Geometry check sheet. Reference: the model listing, model coordinates, mm. A direction names the side the tool comes from. Round coordinates to 2 decimals unless told otherwise and drop trailing zeros. Loops run counter-clockwise (first coordinate to the right, second up) from the corner with the lowest first, then second, coordinate; pieces in that order, holes last. Notation, with made-up numbers: (72.5, 50) -> (111.5, 50) arc R15 cw to (111.5, 70) -> close; hole circle Ø8 at (-2, -8). An arc over 180 degrees is marked (long way). Use a Markdown table: item, result. Add a question column.
Q1. Sectioned sample at D-D, the plane z = 18.5. Enter the section's corners in (x, y).
Q2. Material ranges on L1, parallel to X at y = 2.25, z = -0.5; L2, parallel to X at y = 7, z = -0.5; L3, parallel to Z at x = -19, y = 7, recorded low to high.
Q3. Release check for a two-part mould opening along X. For faces 1 (the face through (-21, 1, -28)), 2 (the face through (-23, 0, 7)), 3 (the face through (24, 6, -5)) record: released by +X, released by -X, zero draft, split by the parting line, or undercut.
Q4. Set-up check for faces 4 (the face through (5, 6, -24)), 5 (the face through (-26, 2.5, -16)): record each of +Z, -Z, +X, -X, +Y, -Y from which the full face is reachable in a straight line by a thin tool's end or side.
Q5. Sectioned sample at B-B, the plane x = 0. Enter the section's corners in (y, z), then the cut area to 3 significant figures.
Q6. Sectioned sample at C-C, the plane y = 4.25. Enter the section's corners in (x, z), then the cut area to 3 significant figures.
Q7. Gauge pin test, flat ends, axial feed: P1, Ø3.5, axis at x = -24.5, y = 5, coming from the -Z side; P2, Ø2, axis at y = 7, z = -23, coming from the -X side; P3, Ø5, axis at y = 4, z = -0.5, coming from the -X side; P4, Ø8, axis at x = 14, z = -11.5, coming from the -Y side. Record the tip position at first contact, or that the pin passes through.
Q8. Sectioned sample at A-A, the plane z = 0. Enter the section's corners in (x, y).
```python
from build123d import *

# Parameters (mm, degrees)
SKETCH1_R           = 35
SKETCH1_R_2         = 22.5
BOSS_EXTRUDE1_DEPTH = 2.5
SKETCH2_R           = 29.5
SKETCH2_R_2         = 22.5
BOSS_EXTRUDE2_DEPTH = 10
CUT_EXTRUDE1_DEPTH  = 52.051444642
SKETCH4_R           = 1.75
CUT_EXTRUDE2_DEPTH  = 52.051444642


with BuildPart() as part:
    # Sketch1 → Boss-Extrude1 (new body)
    with BuildSketch(Plane(origin=(0, 0, 0), x_dir=(1, 0, 0), z_dir=(0, 1, 0))):
        with Locations(Location((0, 0, 0), (0, 0, 270))):
            Circle(SKETCH1_R)
        with Locations(Location((0, 0, 0), (0, 0, 270))):
            Circle(SKETCH1_R_2, mode=Mode.SUBTRACT)
    extrude(amount=BOSS_EXTRUDE1_DEPTH)

    # Sketch2 → Boss-Extrude2 (add)
    with BuildSketch(Plane(origin=(0, 2.5, 0), x_dir=(1, 0, 0), z_dir=(0, 1, 0))):
        with Locations(Location((0, 0, 0), (0, 0, 270))):
            Circle(SKETCH2_R)
        with Locations(Location((0, 0, 0), (0, 0, 270))):
            Circle(SKETCH2_R_2, mode=Mode.SUBTRACT)
    extrude(amount=BOSS_EXTRUDE2_DEPTH)

    # Sketch3 → Cut-Extrude1 (cut, through all)
    with BuildSketch(Plane(origin=(0, 12.5, 0), x_dir=(1, 0, 0), z_dir=(0, 1, 0))):
        with BuildLine():
            Line((-5, 21.937410968), (-5, 26))
            Line((-5, 26), (5, 26))
            Line((5, 26), (5, 21.937410968))
            ThreePointArc((5, 21.937410968), (15.909902577, 15.909902577), (21.937410968, 5))
            Line((21.937410968, 5), (26, 5))
            Line((26, 5), (26, -5))
            Line((26, -5), (21.937410968, -5))
            ThreePointArc((21.937410968, -5), (15.909902577, -15.909902577), (5, -21.937410968))
            Line((5, -21.937410968), (5, -26))
            Line((5, -26), (-5, -26))
            Line((-5, -26), (-5, -21.937410968))
            ThreePointArc((-5, -21.937410968), (-15.909902577, -15.909902577), (-21.937410968, -5))
            Line((-21.937410968, -5), (-26, -5))
            Line((-26, -5), (-26, 5))
            Line((-26, 5), (-21.937410968, 5))
            ThreePointArc((-21.937410968, 5), (-15.909902577, 15.909902577), (-5, 21.937410968))
        make_face()
    extrude(amount=-CUT_EXTRUDE1_DEPTH, mode=Mode.SUBTRACT)

    # Sketch4 → Cut-Extrude2 (cut, through all)
    with BuildSketch(Plane(origin=(0, 12.5, 0), x_dir=(1, 0, 0), z_dir=(0, 1, 0))):
        with Locations(Location((-18.384776311, -18.384776311, 0), (0, 0, 270))):
            Circle(SKETCH4_R)
        with Locations(Location((-18.384776311, 18.384776311, 0), (0, 0, 270))):
            Circle(SKETCH4_R)
        with Locations(Location((18.384776311, 18.384776311, 0), (0, 0, 270))):
            Circle(SKETCH4_R)
        with Locations(Location((18.384776311, -18.384776311, 0), (0, 0, 270))):
            Circle(SKETCH4_R)
    extrude(amount=-CUT_EXTRUDE2_DEPTH, mode=Mode.SUBTRACT)


solid = part.part
```
Values:
| question | item | result |
|---|---|---|
| 1 | outline | (-29.71, 0) -> (-20.13, 0) -> (-20.13, 12.5) -> (-22.98, 12.5) -> (-22.98, 2.5) -> (-29.71, 2.5) -> close; (-16.64, 0) -> (-12.81, 0) -> (-12.81, 12.5) -> (-16.64, 12.5) -> close; (12.81, 0) -> (16.64, 0) -> (16.64, 12.5) -> (12.81, 12.5) -> close; (20.13, 0) -> (29.71, 0) -> (29.71, 2.5) -> (22.98, 2.5) -> (22.98, 12.5) -> (20.13, 12.5) -> close |
| 2 | L1 | -35 to -26, 26 to 35 |
| 2 | L2 | -29.5 to -26, 26 to 29.5 |
| 2 | L3 | -22.57 to -20.02, -16.75 to -12.05, 12.05 to 16.75, 20.02 to 22.57 |
| 3 | face 1 | split by the parting line |
| 3 | face 2 | zero draft |
| 3 | face 3 | undercut |
| 4 | face 4 | +Y, -Y |
| 4 | face 5 | +Y |
| 5 | outline | (0, -35) -> (2.5, -35) -> (2.5, -29.5) -> (12.5, -29.5) -> (12.5, -26) -> (0, -26) -> close; (0, 26) -> (12.5, 26) -> (12.5, 29.5) -> (2.5, 29.5) -> (2.5, 35) -> (0, 35) -> close |
| 5 | area | 115 mm^2 |
| 6 | outline | circle Ø59 at (0, 0); hole (-26, -5) -> (-21.94, -5) arc R22.5 ccw to (-5, -21.94) -> (-5, -26) -> (5, -26) -> (5, -21.94) arc R22.5 ccw to (21.94, -5) -> (26, -5) -> (26, 5) -> (21.94, 5) arc R22.5 ccw to (5, 21.94) -> (5, 26) -> (-5, 26) -> (-5, 21.94) arc R22.5 ccw to (-21.94, 5) -> (-26, 5) -> close; hole circle Ø3.5 at (-18.38, -18.38); hole circle Ø3.5 at (-18.38, 18.38); hole circle Ø3.5 at (18.38, -18.38); hole circle Ø3.5 at (18.38, 18.38) |
| 6 | area | 958 mm^2 |
| 7 | P1 | z = -18.78 |
| 7 | P2 | x = -19.65 |
| 7 | P3 | x = -35 |
| 7 | P4 | through |
| 8 | outline | (-35, 0) -> (-26, 0) -> (-26, 12.5) -> (-29.5, 12.5) -> (-29.5, 2.5) -> (-35, 2.5) -> close; (26, 0) -> (35, 0) -> (35, 2.5) -> (29.5, 2.5) -> (29.5, 12.5) -> (26, 12.5) -> close |
